Design review of the part built by this model. Coordinates are the model's own, in mm. A direction names the side the tool comes from. Round coordinates to 2 decimals unless told otherwise and drop trailing zeros. Order: outer loops, then holes, each group sorted by start corner. A loop starts at its lowest first (then second) coordinate and runs counter-clockwise, first axis right, second up. Notation, with made-up numbers: (4.5, 43) - (60.5, 43) arc R14 cw to (60.5, 70) - close; hole circle Ø8 at (-3, -35). An arc over 180 degrees is marked (long way). Write item = value, one per line.
from build123d import *

# Parameters (mm, degrees)
BOSS_EXTRUDE1_START = 18.4
SKETCH1_W           = 45
SKETCH1_H           = 64
BOSS_EXTRUDE1_DEPTH = 0.8
BOSS_EXTRUDE2_START = 24.2
SKETCH2_W           = 34
SKETCH2_H           = 54
BOSS_EXTRUDE2_DEPTH = 5


with BuildPart() as part:
    # Sketch1 → Boss-Extrude1 (new, symmetric)
    with BuildSketch(Plane.XY.offset(BOSS_EXTRUDE1_START)):
        with Locations((-75, 0)):
            Rectangle(SKETCH1_W, SKETCH1_H)
    extrude(amount=BOSS_EXTRUDE1_DEPTH, both=True)

    # Sketch2 → Boss-Extrude2 (add, symmetric)
    with BuildSketch(Plane.XY.offset(BOSS_EXTRUDE2_START)):
        with Locations((-75, 0)):
            Rectangle(SKETCH2_W, SKETCH2_H)
    extrude(amount=BOSS_EXTRUDE2_DEPTH, both=True)


solid = part.part
1) We need section A-A on y = 19.5. Write out the cut boundary in (x, z), and give its area (3 significant figures).
Findings:
outline = (-97.5, 17.6) - (-52.5, 17.6) - (-52.5, 19.2) - (-58, 19.2) - (-58, 29.2) - (-92, 29.2) - (-92, 19.2) - (-97.5, 19.2) - close
area = 412 mm^2
2) We need section C-C on z = 21.5. Write out the cut boundary in (x, y).
Findings:
outline = (-92, -27) - (-58, -27) - (-58, 27) - (-92, 27) - close
3) Clearance check with flat-ended pins moving along their axes: pin 1 Ø3 at (y, z) = (-14, 26.5) entering from +X; pin 2 Ø3 at (y, z) = (-2, 22) entering from -X; pin 3 Ø5 at (x, z) = (-74, 25.5) entering from -Y. State where each tip first meets the part, or that it passes through.
Findings:
pin_1 = -58
pin_2 = -92
pin_3 = -27
4) To check wall thickness, follow L1, parallel to Y at x = -81, z = 24.5; L2, parallel to X at y = -19.5, z = 20.5; L3, parallel to Z at x = -56, y = 3.5. State the ranges of each line that lie inside material, in increasing order. Write a range as from..to.
Findings:
L1 = -27..27
L2 = -92..-58
L3 = 17.6..19.2
5) For faces 1 (the flat face through (-92, 0, 24)), 2 (the flat face through (-75, 27, 24)), 3 (the flat face through (-75, -27, 24)), list the 3-axis set-ups (+Z, -Z, +X, -X, +Y, -Y) from which the entire face can be reached by the end or side of a thin tool; tool diameter is ignored.
Findings:
face_1 = +Z, -X, +Y, -Y
face_2 = +Z, +X, -X, +Y
face_3 = +Z, +X, -X, -Y
6) We need section D-D on y = -28. Write out the cut boundary in (x, z).
Findings:
outline = (-97.5, 17.6) - (-52.5, 17.6) - (-52.5, 19.2) - (-97.5, 19.2) - close
7) We need section B-B on x = -76.5. Write out the cut boundary in (y, z), and give its area (3 significant figures).
Findings:
outline = (-32, 17.6) - (32, 17.6) - (32, 19.2) - (27, 19.2) - (27, 29.2) - (-27, 29.2) - (-27, 19.2) - (-32, 19.2) - close
area = 642 mm^2
